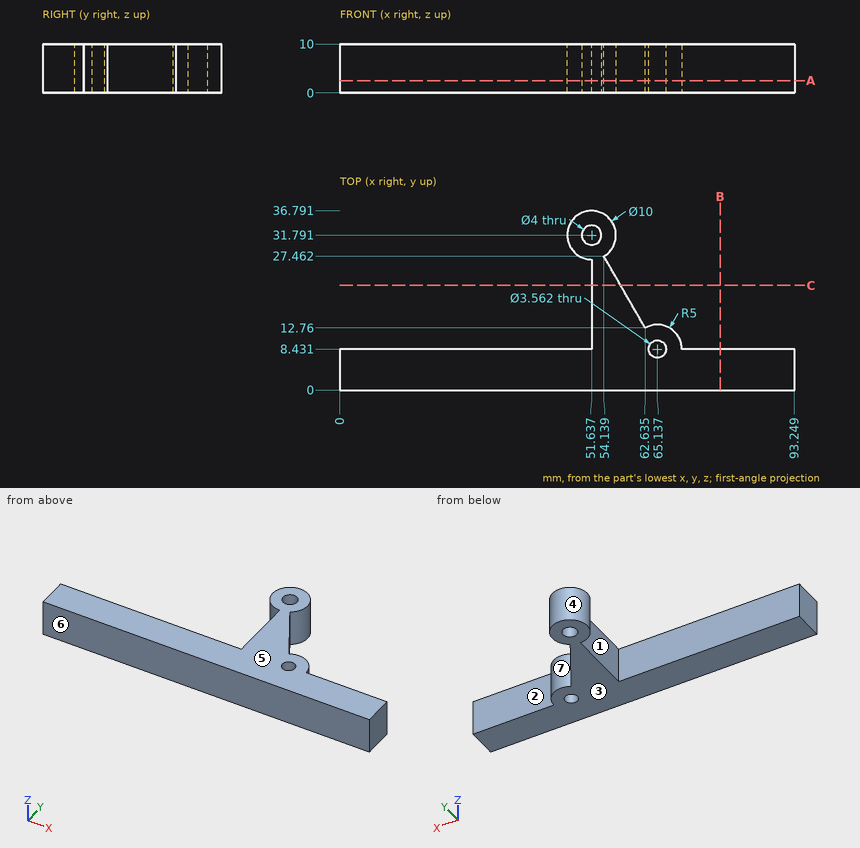
For this review, use the dimensioned drawing (mm, ordinates from the lowest corner) and the shaded views. A direction names the side the tool comes from. Give positions to 0.01 mm unless a question says otherwise; leave off trailing zeros. Write each loop counter-clockwise with the first axis right and the second up, starting at its lowest first coordinate (ties: lowest second). Pieces come first, ordered by that corner, then holes.
(1) Consider section C-C, the plane y = 21.5. Give the boundary of the cut face in (x, z) (1 decimal).
(2) The part is to be moulded in two halves that separate along Y. For the marked faces 4, 5, 6 and 7, say which applies: released by +Y, released by -Y, zero draft, split by the parting line, or undercut.
(3) To check wall thickness, follow L1, parallel to X at y = 8.5, z = 7; L2, parallel to X at y = 33, z = 1 (1 decimal); L3, parallel to Y at x = 52.5, z = 6.5 (1 decimal). State the ranges of each line that lie inside material, in increasing order.
(4) Consider section A-A, the plane z = 2.5. Give the number of separate pieces and of enclosed holes in the cut face, and give its area (3 significant figures).
(5) Consider section B-B, the plane x = 78. Give the boundary of the cut face in (y, z).
(6) For P1, Ø10, axis at x = 57, y = 22.5, coming from the -Z side; P2, Ø3, axis at y = 20, z = 4.5, coming from the -X side; P3, Ø3, axis at x = 79, z = 2.5, coming from the +Y side, all flat-tipped, find the tip position at first contact; note any pin that passes through.
(7) Tool access review of the marked faces 1, 2 and 3: name each direction out of +Z, -Z, +X, -X, +Y, -Y from which nothing blocks a thin tool from reaching the whole face with its end or side.
Returned:
1. outline: (51.6, 0) - (57.6, 0) - (57.6, 10) - (51.6, 10) - close
2. face 4: undercut
2. face 5: zero draft
2. face 6: released by -Y
2. face 7: released by +Y
3. L1: x = 51.64 to 63.36, 66.92 to 70.14
3. L2: x = 46.8 to 50, 53.2 to 56.5
3. L3: y = 0 to 30, 33.6 to 36.7
4. separate pieces: 1
4. enclosed holes: 2
4. area: 1,020 mm2
5. outline: (0, 0) - (8.43, 0) - (8.43, 10) - (0, 10) - close
6. P1: stops at z = 0
6. P2: stops at x = 51.64
6. P3: stops at y = 8.43
7. face 1: +Z, -Z, -X
7. face 2: +Z, -Z, +X, +Y
7. face 3: -Z, +X, -X, +Y, -Y
